Verification items for the finished model (mm, model axes). Coordinates: 2 decimals unless noted, no trailing zeros. Write each loop counter-clockwise with the first axis right and the second up, starting at its lowest first coordinate (ties: lowest second). Pieces come first, ordered by that corner, then holes. Notation, with made-up numbers: (73.25, 2) -> (83.25, 2) arc R23 ccw to (83.25, 26) -> close; hole circle Ø10 at (-30.75, 23). An arc over 180 degrees is marked (long way). Write item = value, one per line. Start each with the question number.
(1) Gauge pin test, flat ends, axial feed: pin 1 Ø1.5 at (x, z) = (-7, 49) entering from -Y; pin 2 Ø1 at (y, z) = (-0.5, 48) entering from +X. Record the tip position at first contact, or that the pin passes through.
(2) Section check B-B (z = 62.5). Record the cut outline in (x, y).
(3) Material ranges on probe 1 along X at (y, z) = (1.35, 36.5); probe 2 along Y at (x, z) = (-5.1, 56); probe 3 along X at (y, z) = (0.25, 67.5), recorded low to high. Write a range as [from, to].
(4) Section check A-A (z = 3). Record the cut outline in (x, y).
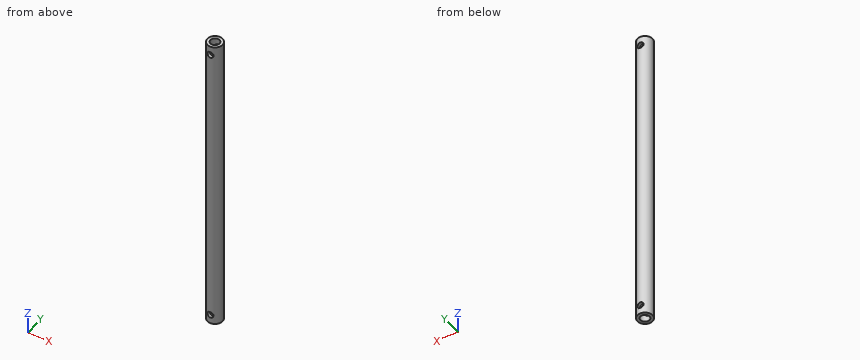
```python
from build123d import *

# Parameters (mm, degrees)
ESQUISSE1_R             = 2.5
ESQUISSE1_R_2           = 1.5
BOSS_EXTRU_1_DEPTH      = 100
ESQUISSE2_R             = 1
ENL_V_MAT_EXTRU_1_DEPTH = 101.399348663


with BuildPart() as part:
    # Esquisse1 → Boss.-Extru.1 (new body)
    with BuildSketch(Plane.XY):
        with Locations((-4.918167702, 1.104491281)):
            Circle(ESQUISSE1_R)
        with Locations((-4.918167702, 1.104491281)):
            Circle(ESQUISSE1_R_2, mode=Mode.SUBTRACT)
    extrude(amount=BOSS_EXTRU_1_DEPTH)

    # Esquisse2 → Enlèv. mat.-Extru.1 (cut, through all)
    with BuildSketch(Plane(origin=(0, 3.604491281, 0), x_dir=(1, 0, 0), z_dir=(0, 1, 0))):
        with Locations(Location((-4.918167702, -3, 0), (0, 0, 270))):
            Circle(ESQUISSE2_R)
        with Locations(Location((-4.918167702, -97, 0), (0, 0, 270))):
            Circle(ESQUISSE2_R)
    extrude(amount=-ENL_V_MAT_EXTRU_1_DEPTH, mode=Mode.SUBTRACT)


solid = part.part
```
Response:
q1.pin_1 = -1.01
q1.pin_2 = -2.68
q2.outline = circle Ø5 at (-4.92, 1.1); hole circle Ø3 at (-4.92, 1.1)
q3.probe_1 = [-7.41, -6.4], [-3.44, -2.43]
q3.probe_2 = [-1.39, -0.38], [2.59, 3.6]
q3.probe_3 = [-7.27, -6.15], [-3.69, -2.57]
q4.outline = (-5.92, -1.19) -> (-5.92, -0.01) arc R1.5 cw to (-5.92, 2.22) -> (-5.92, 3.4) arc R2.5 ccw to start; (-3.92, -1.19) arc R2.5 ccw to (-3.92, 3.4) -> (-3.92, 2.22) arc R1.5 cw to (-3.92, -0.01) -> close
